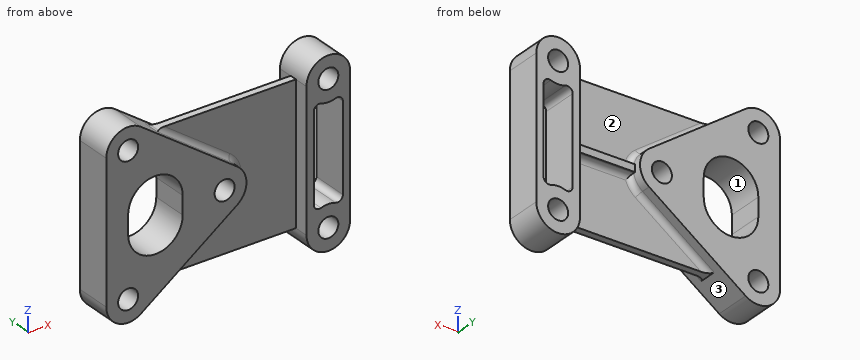
from build123d import *

# Parameters (mm, degrees)
SKETCH1_R             = 5.5
BOSS_EXTRUDE1_DEPTH   = 10
BOSS_EXTRUDE1_2_DEPTH = 10
BOSS_EXTRUDE2_DEPTH   = 2
BOSS_EXTRUDE3_START   = 4
BOSS_EXTRUDE3_DEPTH   = 4
CUT_EXTRUDE1_DEPTH    = 145.416065588
FILLET1_R             = 3
FILLET2_R             = 3
CUT_EXTRUDE2_DEPTH    = 145.416065588


with BuildPart() as part:
    # Sketch1 → Boss-Extrude1 (new, symmetric)
    with BuildSketch(Plane(origin=(0, 0, 0), x_dir=(1, 0, 0), z_dir=(0, 1, 0))):
        with BuildLine():
            Line((0, 38), (0, -38))
            ThreePointArc((0, -38), (6.518533014, -48.67490139), (18.99225328, -47.752353258))
            Line((18.99225328, -47.752353258), (71.99225328, -9.752353258))
            ThreePointArc((71.99225328, -9.752353258), (77, 0), (71.99225328, 9.752353258))
            Line((71.99225328, 9.752353258), (18.99225328, 47.752353258))
            ThreePointArc((18.99225328, 47.752353258), (6.518533014, 48.67490139), (0, 38))
        make_face()
        with Locations(Location((12, 38, 0), (0, 0, 270))):
            Circle(SKETCH1_R, mode=Mode.SUBTRACT)
        with Locations(Location((12, -38, 0), (0, 0, 270))):
            Circle(SKETCH1_R, mode=Mode.SUBTRACT)
        with Locations(Location((65, 0, 0), (0, 0, 270))):
            Circle(SKETCH1_R, mode=Mode.SUBTRACT)
    extrude(amount=BOSS_EXTRUDE1_DEPTH, both=True)



with BuildPart() as body_2:
    # Sketch1 → Boss-Extrude1 2 (new, symmetric)
    with BuildSketch(Plane(origin=(0, 0, 0), x_dir=(1, 0, 0), z_dir=(0, 1, 0))):
        with BuildLine():
            Line((134, 38), (134, -38))
            ThreePointArc((134, -38), (122, -50), (110, -38))
            Line((110, -38), (110, 38))
            ThreePointArc((110, 38), (122, 50), (134, 38))
        make_face()
        with Locations(Location((122, 38, 0), (0, 0, 270))):
            Circle(SKETCH1_R, mode=Mode.SUBTRACT)
        with Locations(Location((122, -38, 0), (0, 0, 270))):
            Circle(SKETCH1_R, mode=Mode.SUBTRACT)
    extrude(amount=BOSS_EXTRUDE1_2_DEPTH, both=True)


with BuildPart() as part_1:
    add(part.part)

    add(body_2.part)  # Boss-Extrude2 merges body 2
    # Sketch2 → Boss-Extrude2 (add, symmetric)
    with BuildSketch(Plane(origin=(0, 0, 0), x_dir=(1, 0, 0), z_dir=(0, 1, 0))):
        with BuildLine():
            Line((110, 38), (110, -38))
            Line((110, -38), (32.594219666, -38))
            Line((32.594219666, -38), (71.99225328, -9.752353258))
            ThreePointArc((71.99225328, -9.752353258), (77, 0), (71.99225328, 9.752353258))
            Line((71.99225328, 9.752353258), (32.594219666, 38))
            Line((32.594219666, 38), (110, 38))
        make_face()
    extrude(amount=BOSS_EXTRUDE2_DEPTH, both=True)

    # Sketch3 → Boss-Extrude3 (add)
    with BuildSketch(Plane(origin=(0, 2, 0), x_dir=(1, 0, 0), z_dir=(0, 1, 0)).offset(BOSS_EXTRUDE3_START)):
        with BuildLine():
            Line((76.832159566, 2), (110, 2))
            Line((110, 2), (110, -2))
            Line((110, -2), (76.832159566, -2))
            ThreePointArc((76.832159566, -2), (77, 0), (76.832159566, 2))
        make_face()
    extrude(amount=-BOSS_EXTRUDE3_DEPTH)

    # Sketch4 → Cut-Extrude1 (cut, through all)
    with BuildSketch(Plane(origin=(0, 10, 0), x_dir=(1, 0, 0), z_dir=(0, 1, 0))):
        with BuildLine():
            Line((114, 29.05572809), (114, -29.05572809))
            ThreePointArc((114, -29.05572809), (122, -26), (130, -29.05572809))
            Line((130, -29.05572809), (130, 29.05572809))
            ThreePointArc((130, 29.05572809), (122, 26), (114, 29.05572809))
        make_face()
    extrude(amount=-CUT_EXTRUDE1_DEPTH, mode=Mode.SUBTRACT)

    # Fillet1
    fillet1_edges = [part_1.edges().sort_by_distance(p)[0] for p in [
        (114, 0, -29.05572809),
        (130, 0, -29.05572809),
        (130, 0, 29.05572809),
        (114, 0, 29.05572809),
    ]]
    fillet(fillet1_edges, radius=FILLET1_R)

    # Fillet2
    fillet2_edges = [part_1.edges().sort_by_distance(p)[0] for p in [
        (52.293236473, -2, -23.876176629),
        (77, -2, 0),
        (52.293236473, -2, 23.876176629),
        (32.594219666, 0, 38),
        (52.293236473, 2, -23.876176629),
        (75.179114648, 2, -6.354968528),
        (52.293236473, 2, 23.876176629),
        (75.179114648, 2, 6.354968528),
        (93.416079783, 2, 2),
        (93.416079783, 2, -2),
    ]]
    fillet(fillet2_edges, radius=FILLET2_R)

    # Sketch5 → Cut-Extrude2 (cut, through all)
    with BuildSketch(Plane(origin=(0, 10, 0), x_dir=(1, 0, 0), z_dir=(0, 1, 0))):
        with BuildLine():
            Line((41.999381369, 5.001855509), (42.000618401, -4.998144414))
            ThreePointArc((42.000618401, -4.998144414), (27.002474063, -19.999999847), (12.000618631, -5.001855509))
            Line((12.000618631, -5.001855509), (11.999381599, 4.998144414))
            ThreePointArc((11.999381599, 4.998144414), (26.997525937, 19.999999847), (41.999381369, 5.001855509))
        make_face()
    extrude(amount=-CUT_EXTRUDE2_DEPTH, mode=Mode.SUBTRACT)


solid = part_1.part
CAD build for the part. Positions are in the model's coordinates, mm. Face numbers are marked on the shaded views. A direction names the side the tool comes from. Round coordinates to 2 decimals unless told otherwise and drop trailing zeros. Write each loop counter-clockwise with the first axis right and the second up, starting at its lowest first coordinate (ties: lowest second). Pieces come first, ordered by that corner, then holes. Notation, with made-up numbers: (52.25, 68.25) -> (110.25, 68.25) arc R18 cw to (110.25, 91.25) -> close; hole circle Ø7 at (-10.75, 1.5). An arc over 180 degrees is marked (long way). Answer as a JSON object with one key per item and string values.
(1) Band-saw the part on D-D, the plane x = 20.5. List the corners of the cut face in (y, z).
Reported:
{"outline": "(-10, -46.67) -> (10, -46.67) -> (10, -18.52) -> (-10, -18.52) -> close; (-10, 18.52) -> (10, 18.52) -> (10, 46.67) -> (-10, 46.67) -> close"}
(2) Band-saw the part on C-C, the plane y = 0. List the corners of the cut face in (x, z), then the cut area to 3 significant figures.
Reported:
{"outline": "(0, -38) arc R12 ccw to (18.99, -47.75) -> (32.59, -38) -> (110, -38) arc R12 ccw to (134, -38) -> (134, 38) arc R12 ccw to (110, 38) -> (33.56, 38) arc R3 cw to (31.81, 38.56) -> (18.99, 47.75) arc R12 ccw to (0, 38) -> close; hole circle Ø11 at (12, -38); hole circle Ø11 at (12, 38); hole (12, -5) arc R15 ccw to (42, -5) -> (42, 5) arc R15 ccw to (12, 5) -> close; hole circle Ø11 at (65, 0); hole (114, -23.86) arc R3 ccw to (118, -26.69) arc R12 cw to (126, -26.69) arc R3 ccw to (130, -23.86) -> (130, 23.86) arc R3 ccw to (126, 26.69) arc R12 cw to (118, 26.69) arc R3 ccw to (114, 23.86) -> close; hole circle Ø11 at (122, -38); hole circle Ø11 at (122, 38)", "area": "8,830 mm^2"}
(3) Which spindle directions (+Z, -Z, +X, -X, +Y, -Y) get a long thin tool onto all of the face, cutting with end or side? Do the marked faces 1, 2 and 3. Say none if no direction does.
Reported:
{"face 1": "+Y, -Y", "face 2": "+Z, +Y", "face 3": "-Z"}
(4) Band-saw the part on B-B, the plane z = 0. List the corners of the cut face in (x, y), then the cut area to 3 significant figures.
Reported:
{"outline": "(0, -10) -> (12, -10) -> (12, 10) -> (0, 10) -> close; (42, -10) -> (59.5, -10) -> (59.5, 10) -> (42, 10) -> close; (70.5, -10) -> (77, -10) -> (77, -5) arc R3 cw to (80, -2) -> (110, -2) -> (110, -10) -> (114, -10) -> (114, 10) -> (110, 10) -> (110, 6) -> (77, 6) -> (77, 10) -> (70.5, 10) -> close; (130, -10) -> (134, -10) -> (134, 10) -> (130, 10) -> close", "area": "1,150 mm^2"}
(5) Probe probe 1 along X at (y, z) = (0.5, 0); probe 2 along X at (y, z) = (-3.5, 0); probe 3 along X at (y, z) = (7, 2). List the from-to ranges inside material, lowest first. Write a range as [from, to].
Reported:
{"probe 1": "x = [0, 12], [42, 59.5], [70.5, 114], [130, 134]", "probe 2": "x = [0, 12], [42, 59.5], [70.5, 77.4], [110, 114], [130, 134]", "probe 3": "x = [0, 12], [42, 59.88], [70.12, 76.83], [110, 114], [130, 134]"}
(6) Pin check, flat tips, straight feed: P1, Ø2, axis at x = 93.5, z = -0.5, coming from the +Y side; P2, Ø8, axis at x = 50.5, y = 7, coming from the +Z side; P3, Ø5, axis at x = 116.5, y = 3.5, coming from the +Z side; P4, Ø10, axis at x = 12, z = -38, coming from the +Y side. Stop position of each tip, or through.
Reported:
{"P1": "stops at y = 6", "P2": "stops at z = 28.03", "P3": "stops at z = 49.62", "P4": "passes through"}
(7) Band-saw the part on A-A, the plane y = -7.5. Count the separate pieces of the cut face and the enclosed holes in it, then the cut area to 3 significant figures.
Reported:
{"separate pieces": "2", "enclosed holes": "7", "area": "4,900 mm^2"}
